from build123d import *

# Parameters (mm, degrees)
EXTRUDE_1_DEPTH     = 58
SKETCH_2_R          = 4.25
CUT_EXTRUDE_1_DEPTH = 58.5
SKETCH_3_R          = 4.25
CUT_EXTRUDE_2_DEPTH = 58.5
EXTRUDE_2_DEPTH     = 3.2
EXTRUDE_3_DEPTH     = 3.2
FILLET_1_R          = 2


with BuildPart() as part:
    # 草图1 → 凸台-拉伸1 (new body)
    with BuildSketch(Plane.XY):
        Polygon((0, 58), (0, 0), (58, 0), (58, 5.5), (5.5, 5.5), (5.5, 58), align=None)
    extrude(amount=EXTRUDE_1_DEPTH)

    # 草图2 → 切除-拉伸1 (cut)
    with BuildSketch(Plane.XZ):
        with Locations(Location((43.5, 44, 0), (0, 0, 270))):
            Circle(SKETCH_2_R)
        with Locations((43.5, 14)):
            Circle(SKETCH_2_R)
        with BuildLine():
            Line((19, 48.25), (29, 48.25))
            ThreePointArc((29, 48.25), (33.25, 44), (29, 39.75))
            Line((29, 39.75), (19, 39.75))
            ThreePointArc((19, 39.75), (14.75, 44), (19, 48.25))
        make_face()
        with BuildLine():
            Line((19, 9.75), (29, 9.75))
            ThreePointArc((29, 9.75), (33.25, 14), (29, 18.25))
            Line((29, 18.25), (19, 18.25))
            ThreePointArc((19, 18.25), (14.75, 14), (19, 9.75))
        make_face()
    extrude(amount=-CUT_EXTRUDE_1_DEPTH, mode=Mode.SUBTRACT)

    # 草图3 → 切除-拉伸2 (cut)
    with BuildSketch(Plane.ZY):
        with Locations(Location((44, 43.5, 0), (0, 0, 270))):
            Circle(SKETCH_3_R)
        with Locations(Location((14, 43.5, 0), (0, 0, 270))):
            Circle(SKETCH_3_R)
        with BuildLine():
            Line((39.75, 29), (39.75, 19))
            ThreePointArc((39.75, 19), (44, 14.75), (48.25, 19))
            Line((48.25, 19), (48.25, 29))
            ThreePointArc((48.25, 29), (44, 33.25), (39.75, 29))
        make_face()
        with BuildLine():
            Line((9.75, 29), (9.75, 19))
            ThreePointArc((9.75, 19), (14, 14.75), (18.25, 19))
            Line((18.25, 19), (18.25, 29))
            ThreePointArc((18.25, 29), (14, 33.25), (9.75, 29))
        make_face()
    extrude(amount=-CUT_EXTRUDE_2_DEPTH, mode=Mode.SUBTRACT)

    # 草图4 → 凸台-拉伸2 (add)
    with BuildSketch(Plane.XY.offset(58)):
        Polygon((5.5, 58), (10.5, 58), (10.5, 53), (53, 10.5), (58, 10.5), (58, 5.5), (5.5, 5.5), align=None)
    extrude(amount=-EXTRUDE_2_DEPTH)

    # 草图5 → 凸台-拉伸3 (add)
    with BuildSketch(Plane(origin=(0, 0, 0), x_dir=(-1, 0, 0), z_dir=(0, 0, -1))):
        Polygon((-10.5, 58), (-10.5, 53), (-53, 10.5), (-58, 10.5), (-58, 5.5), (-5.5, 5.5), (-5.5, 58), align=None)
    extrude(amount=-EXTRUDE_3_DEPTH)

    # 圆角1
    fillet_1_edges = [part.edges().sort_by_distance(p)[0] for p in [
        (10.5, 58, 56.4),
        (10.5, 53, 56.4),
        (53, 10.5, 56.4),
        (58, 10.5, 56.4),
        (10.5, 53, 1.6),
        (10.5, 58, 1.6),
        (58, 10.5, 1.6),
        (53, 10.5, 1.6),
    ]]
    fillet(fillet_1_edges, radius=FILLET_1_R)


solid = part.part
Here's how the part is built. I have some questions about the finished solid (model axes, mm). A direction names the side the tool comes from. Round coordinates to 2 decimals unless told otherwise and drop trailing zeros. Write each loop counter-clockwise with the first axis right and the second up, starting at its lowest first coordinate (ties: lowest second). Pieces come first, ordered by that corner, then holes.
1. Will these pins go through, and if not, where does the flat tip stop? pin 1 Ø6 at (y, z) = (24, 39.5) entering from +X; pin 2 Ø10 at (x, z) = (43.5, 44) entering from -Y; pin 3 Ø2.5 at (x, z) = (55, 2) entering from +Y; pin 4 Ø5 at (x, z) = (26, 52) entering from +Y.
2. If we mould it in two halves opening along Z, with no side actions, what happens to faces 1 (the flat face through (20, 20, 3.2)), 2 (the cylindrical face through (57.43, 9.9, 1.62))? For each: released by +Z, released by -Z, zero draft, split by the parting line, or undercut.
3. Suppose I cut it at C-C (z = 44). List the corners of the cut face in (x, y) for me, and give its area (3 significant figures).
4. For faces 3 (the flat face through (10.5, 55, 56)), 4 (the flat face through (20, 20, 54.8)), 5 (the cylindrical face through (2.71, 14.75, 43.91)), which set-ups out of +Z, -Z, +X, -X, +Y, -Y let a thin tool reach every point of the face, with its end or its side?
5. Suppose I cut it at B-B (y = 22). List the corners of the cut face in (x, z) for me, and give its area (3 significant figures).
6. Suppose I cut it at D-D (x = 51.5). List the corners of the cut face in (y, z) for me, and give its area (3 significant figures).
7. Suppose I cut it at A-A (x = 28). List the corners of the cut face in (y, z) for me.
8. I need wall thicknesses on L1, parallel to X at y = 3.85, z = 44; L2, parallel to Z at x = 8.5, y = 14; L3, parallel to Z at x = 1, y = 43. Which ranges of each line are inside material? Lowest first, please.
Answer sheet:
1. pin 1: stops at x = 5.5
1. pin 2: stops at y = 0
1. pin 3: stops at y = 10.5
1. pin 4: stops at y = 5.5
2. face 1: undercut
2. face 2: zero draft
3. outline: (0, 0) - (14.75, 0) - (14.75, 5.5) - (5.5, 5.5) - (5.5, 14.75) - (0, 14.75) - close; (0, 33.25) - (5.5, 33.25) - (5.5, 39.25) - (0, 39.25) - close; (0, 47.75) - (5.5, 47.75) - (5.5, 58) - (0, 58) - close; (33.25, 0) - (39.25, 0) - (39.25, 5.5) - (33.25, 5.5) - close; (47.75, 0) - (58, 0) - (58, 5.5) - (47.75, 5.5) - close
3. area: 311 mm2
4. face 3: +Z, -Z, +X, +Y
4. face 4: +X, +Y
4. face 5: +X, -X
5. outline: (0, 0) - (41.5, 0) - (41.5, 3.2) - (5.5, 3.2) - (5.5, 9.75) - (0, 9.75) - close; (0, 18.25) - (5.5, 18.25) - (5.5, 39.75) - (0, 39.75) - close; (0, 48.25) - (5.5, 48.25) - (5.5, 54.8) - (41.5, 54.8) - (41.5, 58) - (0, 58) - close
5. area: 456 mm2
6. outline: (0, 0) - (12, 0) - (12, 3.2) - (5.5, 3.2) - (5.5, 54.8) - (12, 54.8) - (12, 58) - (0, 58) - close
6. area: 361 mm2
7. outline: (0, 0) - (35.5, 0) - (35.5, 3.2) - (5.5, 3.2) - (5.5, 9.75) - (0, 9.75) - close; (0, 18.25) - (5.5, 18.25) - (5.5, 39.75) - (0, 39.75) - close; (0, 48.25) - (5.5, 48.25) - (5.5, 54.8) - (35.5, 54.8) - (35.5, 58) - (0, 58) - close
8. L1: x = 0 to 14.75, 33.25 to 39.25, 47.75 to 58
8. L2: z = 0 to 3.2, 54.8 to 58
8. L3: z = 0 to 9.78, 18.22 to 39.78, 48.22 to 58
